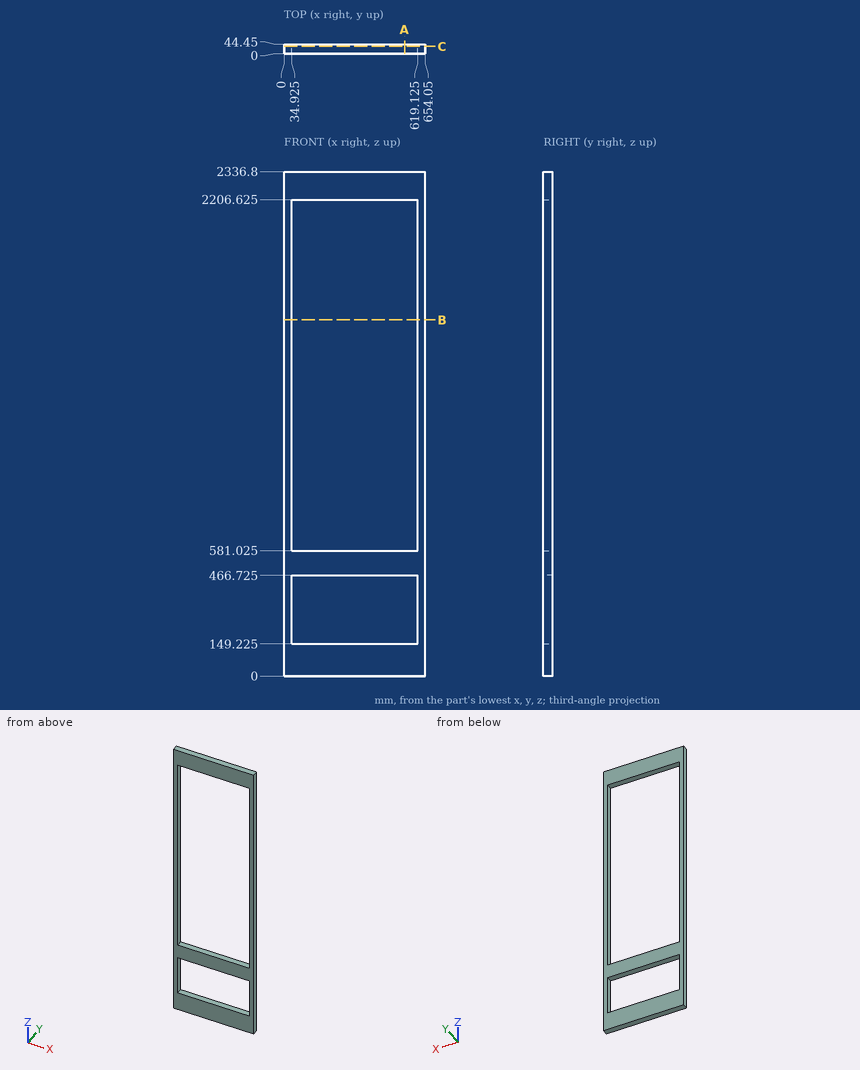
Geometry: see drawing. Coordinates: mm, zero at the bounding-box minimum. Coordinates: 2 decimals unless noted, no trailing zeros. Loops run counter-clockwise (first coordinate to the right, second up) from the corner with the lowest first, then second, coordinate; pieces in that order, holes last.
Q1. Material intervals for line 1 (Z direction, x = 326, y = 5.5) (3 decimals); line 2 (X direction, y = 27.5, z = 2137) (3 decimals), sorted ascending.
Q2. Cut plane A-A (x = 558.5). Output: boundary loops of the cut face in (y, z) (3 decimals).
Q3. Cut plane C-C (y = 33). Output: boundary loops of the cut face in (x, z) (3 decimals).
Q4. Cut plane B-B (z = 1649.5). Output: boundary loops of the cut face in (x, y) (3 decimals), then the cut area to 3 significant figures.
Working result:
1. line 1: z = 0 to 149.225, 466.725 to 581.025, 2206.625 to 2336.8
1. line 2: x = 0 to 34.925, 619.125 to 654.05
2. outline: (0, 0) - (44.45, 0) - (44.45, 149.225) - (0, 149.225) - close; (0, 466.725) - (44.45, 466.725) - (44.45, 581.025) - (0, 581.025) - close; (0, 2206.625) - (44.45, 2206.625) - (44.45, 2336.8) - (0, 2336.8) - close
3. outline: (0, 0) - (654.05, 0) - (654.05, 2336.8) - (0, 2336.8) - close; hole (34.925, 149.225) - (619.125, 149.225) - (619.125, 466.725) - (34.925, 466.725) - close; hole (34.925, 581.025) - (619.125, 581.025) - (619.125, 2206.625) - (34.925, 2206.625) - close
4. outline: (0, 0) - (34.925, 0) - (34.925, 44.45) - (0, 44.45) - close; (619.125, 0) - (654.05, 0) - (654.05, 44.45) - (619.125, 44.45) - close
4. area: 3,100 mm2
